from build123d import *

# Parameters (mm, degrees)
SKETCH1_R           = 8
BOSS_EXTRUDE1_DEPTH = 20


with BuildPart() as part:
    # Sketch1 → Boss-Extrude1 (new body)
    with BuildSketch(Plane(origin=(0, 0, 0), x_dir=(0, 0, -1), z_dir=(1, 0, 0))):
        with BuildLine():
            Line((-139.248116041, 30.619697735), (-101.955216425, 90.044413341))
            ThreePointArc((-101.955216425, 90.044413341), (-94.694061218, 96.914975381), (-85.014811773, 99.413200323))
            Line((-85.014811773, 99.413200323), (33.441717862, 99.413200323))
            ThreePointArc((33.441717862, 99.413200323), (43.441717862, 96.733708398), (50.762225937, 89.413200323))
            Line((50.762225937, 89.413200323), (85.840913151, 28.655131806))
            ThreePointArc((85.840913151, 28.655131806), (85.840913151, 18.655131806), (77.180659113, 13.655131806))
            Line((77.180659113, 13.655131806), (54.086648345, 13.655131806))
            ThreePointArc((54.086648345, 13.655131806), (49.086648345, 14.994877768), (45.426394308, 18.655131806))
            Line((45.426394308, 18.655131806), (27.66821517, 49.413200323))
            ThreePointArc((27.66821517, 49.413200323), (20.347707094, 56.733708398), (10.347707094, 59.413200323))
            Line((10.347707094, 59.413200323), (-62.406928949, 59.413200323))
            ThreePointArc((-62.406928949, 59.413200323), (-72.406928949, 56.733708398), (-79.727437025, 49.413200323))
            Line((-79.727437025, 49.413200323), (-96.533588998, 20.304091226))
            ThreePointArc((-96.533588998, 20.304091226), (-100.193843035, 16.643837188), (-105.193843035, 15.304091226))
            Line((-105.193843035, 15.304091226), (-130.777913715, 15.304091226))
            ThreePointArc((-130.777913715, 15.304091226), (-139.528801244, 20.464466504), (-139.248116041, 30.619697735))
        make_face()
        with Locations((-31.553843665, 79.413200323)):
            Circle(SKETCH1_R, mode=Mode.SUBTRACT)
        with Locations((-117.681607113, 30.619697735)):
            Circle(SKETCH1_R, mode=Mode.SUBTRACT)
        with Locations((63.073370123, 28.655131806)):
            Circle(SKETCH1_R, mode=Mode.SUBTRACT)
    extrude(amount=BOSS_EXTRUDE1_DEPTH)


solid = part.part
Build history of the part. All positions in model axes, mm. A direction names the side the tool comes from. Give positions to 0.01 mm unless a question says otherwise; leave off trailing zeros. Order: outer loops, then holes, each group sorted by start corner. A loop starts at its lowest first (then second) coordinate and runs counter-clockwise, first axis right, second up. Notation, with made-up numbers: M 86,48 L 93,48 A19 ccw 93,84 Z; hole C -27.5,18.5 d8. An arc over 180 degrees is marked long. Use one line per item in the form item = value.
Q1. Slice it at C-C, the plane x = 15. Write the cut outline in (y, z).
Conclusion:
outline = M 13.66,-77.18 A10 ccw 28.66,-85.84 L 89.41,-50.76 A20 ccw 99.41,-33.44 L 99.41,85.01 A20 ccw 90.04,101.96 L 30.62,139.25 A10 ccw 15.3,130.78 L 15.3,105.19 A10 ccw 20.3,96.53 L 49.41,79.73 A20 cw 59.41,62.41 L 59.41,-10.35 A20 cw 49.41,-27.67 L 18.66,-45.43 A10 ccw 13.66,-54.09 Z; hole C 28.66,-63.07 d16; hole C 30.62,117.68 d16; hole C 79.41,31.55 d16
Q2. Slice it at B-B, the plane y = 34.5. Write the cut outline in (x, z).
Conclusion:
outline = M 0,-82.47 L 20,-82.47 L 20,-68.54 L 0,-68.54 Z; M 0,-57.61 L 20,-57.61 L 20,-36.28 L 0,-36.28 Z; M 0,88.34 L 20,88.34 L 20,110.69 L 0,110.69 Z; M 0,124.68 L 20,124.68 L 20,136.81 L 0,136.81 Z
Q3. Pin check, flat tips, straight feed: P1, Ø1.5, axis at x = 9.5, y = 24, coming from the +Z side; P2, Ø2, axis at x = 5.5, y = 30, coming from the -Z side; P3, Ø5, axis at x = 7, y = 35.5, coming from the -Z side; P4, Ø12, axis at x = 4.5, y = 28.5, coming from the -Z side. Stop position of each tip, or through.
Conclusion:
P1 = 140.76
P2 = -85.64
P3 = -83.33
P4 = -87.18
Q4. Slice it at D-D, the plane y = 74. Write the cut outline in (x, z).
Conclusion:
outline = M 0,-59.66 L 20,-59.66 L 20,25.66 L 0,25.66 Z; M 0,37.44 L 20,37.44 L 20,112.02 L 0,112.02 Z
Q5. Wall check: probe 1 along Z at (x, y) = (4.75, 25); probe 2 along Z at (x, y) = (16.5, 35.5); probe 3 along Y at (x, z) = (19, 23). Give the ranges that are in metal, low to high.
Conclusion:
probe_1 = -87.09 to -70.19, -55.96 to -41.76, 93.82 to 111.99, 123.38 to 140.77
probe_2 = -81.89 to -67.21, -58.93 to -35.7, 87.76 to 111.34, 124.02 to 136.19
probe_3 = 59.41 to 99.41
Q6. Slice it at A-A, the plane y = 85. Write the cut outline in (x, z).
Conclusion:
outline = M 0,-53.31 L 20,-53.31 L 20,25.83 L 0,25.83 Z; M 0,37.28 L 20,37.28 L 20,105.12 L 0,105.12 Z
Q7. Which spindle directions (+Z, -Z, +X, -X, +Y, -Y) get a long thin tool onto all of the face, cutting with end or side? Do faces 4 (the flat face through (10, 15.304, 118)), 5 (the flat face through (10, 59.413, 26)), 6 (the cylindrical face through (9.86, 71.603, 33.288)). Say none if no direction does.
Conclusion:
face_4 = +Z, +X, -X, -Y
face_5 = +X, -X, -Y
face_6 = +X, -X
Q8. Pull direction Z, two halves, no side cores. Call faces 1 (the cylindrical face through (9.86, 96.846, 94.818)), 2 (the cylindrical face through (9.86, 34.062, -57.177)), 3 (the cylindrical face through (9.86, 96.81, -43.31)): released by +Z, released by -Z, zero draft, split by the parting line, or undercut.
Conclusion:
face_1 = released by +Z
face_2 = undercut
face_3 = released by -Z
